Autodesk Inventor part; units mm, degrees
ref_plane "YZ Plane" through (0, 0, 0) normal (1, 0, 0) x (0, 1, 0)
ref_plane "XZ Plane" through (0, 0, 0) normal (0, 1, 0) x (-1, 0, 0)
ref_plane "XY Plane" through (0, 0, 0) normal (0, 0, 1) x (1, 0, 0)
sketch "Sketch1" plane through (0, 0, 0) normal (0, 0, 1) x (1, 0, 0)
  circle A0 centre (0, 0) radius 39.4843
  dimension "d0" = 78.9686
extrude "Extrusion1" add sketch "Sketch1" along normal blind 218.44
sketch "Sketch2" plane through (0, 0, 0) normal (1, 0, 0) x (0, 1, 0)
  line L0 (39.4843, 0) -> (39.4843, 218.44)
  line L1 (39.4843, 83.5771) -> (39.4843, 128.0271)
  line L2 (39.4843, 128.0271) -> (166.4843, 128.0271)
  line L3 (166.4843, 128.0271) -> (131.3819, 76.4226) construction
  line L4 (131.3819, 76.4226) -> (39.4843, 83.5771) construction
  spline S0 degree 2 poles (166.4843, 128.0271) (131.3819, 76.4226) (39.4843, 83.5771) knots 1 1 1 2 2 2
  line L5 (-39.4843, 83.5747) -> (-39.4843, 128.0271)
  line L6 (-39.4843, 0) -> (-39.4843, 218.44)
  line L7 (-39.4843, 83.5747) -> (-39.4843, 128.0271)
  line L8 (-39.4843, 128.0271) -> (-166.4843, 128.0271)
  line L9 (-166.4843, 128.0271) -> (-149.7384, 83.5714) construction
  line L10 (-149.7384, 83.5714) -> (-39.4843, 83.5747) construction
  spline S1 degree 2 poles (-166.4843, 128.0271) (-149.7384, 83.5714) (-39.4843, 83.5747) knots 1 1 1 2 2 2
  line L11 (-39.4843, 128.0271) -> (48.468, 128.0271)
  line L12 (-39.4843, 83.5747) -> (39.4843, 83.5771)
  line L13 (-54.9885, 128.0271) -> (39.4843, 128.0271)
  line L14 (39.4843, 0) -> (39.4843, 218.44)
  line L15 (-39.4843, 83.5747) -> (39.4843, 83.5771)
  point P0 (0, 0)
  dimension "d3" = 44.45
  dimension "d4" = 127
  dimension "d5" = 127
extrude "Extrusion2" add sketch "Sketch2" along normal blind 3.175
chamfer "Chamfer1" distance 3.175 angle 45 1 edges at (3.175, -102.9204, 128.0271)
chamfer "Chamfer2" distance 3.175 angle 45 1 edges at (3.175, 102.9204, 128.0271)
sketch "Sketch3" plane through (0, 0, 0) normal (0, 1, 0) x (-1, 0, 0)
  line L0 (-39.4843, 0) -> (39.4843, 0)
  line L1 (-33.3888, 0) -> (9.1562, 0)
  line L2 (9.1562, 0) -> (44.2001, -3.3503) construction
  line L3 (44.2001, -3.3503) -> (62.7444, -45.9959) construction
  spline S0 degree 2 poles (9.1562, 0) (44.2001, -3.3503) (62.7444, -45.9959) knots 1 1 1 2 2 2
  line L4 (62.7444, -45.9959) -> (-9.2544, -6.0902) construction
  line L5 (-9.2544, -6.0902) -> (-44.8829, -45.9959) construction
  spline S1 degree 2 poles (62.7444, -45.9959) (-9.2544, -6.0902) (-44.8829, -45.9959) knots 1 1 1 2 2 2
  line L6 (-44.8829, -45.9959) -> (-49.2667, -15.2331) construction
  line L7 (-49.2667, -15.2331) -> (-33.3888, 0) construction
  spline S2 degree 2 poles (-44.8829, -45.9959) (-49.2667, -15.2331) (-33.3888, 0) knots 1 1 1 2 2 2
  point P0 (0, 0)
  dimension "d14" = 42.545
extrude "Extrusion3" add sketch "Sketch3" along normal mid plane 6.35
fillet "Fillet1" radius 3.175 1 edges at (12.1163, 3.175, 0)
fillet "Fillet2" radius 3.175 1 edges at (12.1163, -3.175, 0)
sketch "Sketch4" plane through (0, 0, 218.44) normal (0, 0, 1) x (1, 0, 0)
  point P0 (0, 0)
properties part number "wings"
For this review, take the finished solid that the model builds, in its own axes (mm). A direction names the side the tool comes from. Round coordinates to 2 decimals unless told otherwise and drop trailing zeros. Loops run counter-clockwise (first coordinate to the right, second up) from the corner with the lowest first, then second, coordinate; pieces in that order, holes last.
(1) Wall thickness on line 1 along X through (y, z) = (86, 107) (3 decimals); line 2 along Y through (x, z) = (-1.5, 71.5); line 3 along Y through (x, z) = (4.5, 35): over which ranges is each line inside the solid? List them lowest first.
Returned:
line 1: x = 0 to 3.175
line 2: y = -39.46 to 39.46
line 3: y = -39.23 to 39.23
(2) We need section A-A (z = 137.5). Give the boundary of the cut face in (x, y), plus the area to 3 significant figures.
Returned:
outline: circle Ø78.97 at (0, 0)
area: 4,900 mm2
(3) Clearance check with flat-ended pins moving along their axes: P1, Ø5, axis at x = 7.5, y = 61, coming from the -Z side; P2, Ø13, axis at x = -32.5, z = -25, coming from the -Y side (3 decimals); P3, Ø13.5, axis at y = -119.5, z = 95.5, coming from the -X side; P4, Ø5, axis at x = -21.5, z = 182.5, coming from the +Y side. State where each tip first meets the part, or that it passes through.
Returned:
P1: passes through
P2: stops at y = -3.175
P3: stops at x = 0
P4: stops at y = 34.61
(4) Tool access review of faces 1 (the flat face through (0, 88, 108)), 2 (the flat face through (3.175, -89, 109)), 3 (the flat face through (0, -90, 111)): name each direction out of +Z, -Z, +X, -X, +Y, -Y from which nothing blocks a thin tool from reaching the whole face with its end or side.
Returned:
face 1: +Z, -Z, -X, +Y
face 2: +Z, -Z, +X, -Y
face 3: +Z, -Z, -X, -Y
